Here's how the part is built. I have some questions about the finished solid (model axes, mm). Coordinates: 2 decimals unless noted, no trailing zeros. Write each loop counter-clockwise with the first axis right and the second up, starting at its lowest first coordinate (ties: lowest second). Pieces come first, ordered by that corner, then holes. Notation, with made-up numbers: (33.25, 80) -> (85.25, 80) arc R27 cw to (85.25, 103) -> close; hole circle Ø8 at (4, -9). An arc over 180 degrees is marked (long way). Use a Markdown table: item, result. Add a question column.
Item 1: If I drill on line 1 along Y through (x, z) = (0, 18.5); line 2 along X through (y, z) = (-3, 7.75); line 3 along X through (y, z) = (6, 2), over which ranges is the centre line in solid material (lowest first)? Write a range as from..to.
Item 2: Imagine slicing it at C-C, the plane z = 3. Write out the boundary of the cut face in (x, y).
Item 3: Will these pins go through, and if not, where does the flat tip stop? pin 1 Ø2 at (x, z) = (-12, 12.5) entering from +Y; pin 2 Ø9 at (x, y) = (0, 0) entering from +Z.
Item 4: If we mould it in two halves opening along X, with no side actions, what happens to faces 1 (the flat face through (15, 0, 12)), 2 (the flat face through (-15, 0, 12)), 3 (the flat face through (6, -5, 0)), 4 (the cylindrical face through (-7.493, 0.33, 12.325))? For each: pulls with the +X half, pulls with the -X half, needs draft (parallel to the pull), parting line crosses it, or undercut.
Item 5: Imagine slicing it at B-B, the plane y = 0. Write out the boundary of the cut face in (x, z), and give its area (3 significant figures).
Item 6: Imagine slicing it at A-A, the plane x = 0. Write out the boundary of the cut face in (y, z).
Item 7: Imagine slicing it at D-D, the plane y = -22. Write out the boundary of the cut face in (x, z).
```python
from build123d import *

# Parameters (mm, degrees)
F0_W     = 30
F0_H     = 50
F0_R     = 7.5
F1_DEPTH = 25
F2_SIZE  = 5


with BuildPart() as f1:
    # F0 (on Top) → F1 (new body)
    with BuildSketch(Plane.XY):
        Rectangle(F0_W, F0_H)
        Circle(F0_R, mode=Mode.SUBTRACT)
    extrude(amount=F1_DEPTH)

    # F2
    f2_edges = [f1.edges().sort_by_distance(p)[0] for p in [
        (15, -25, 12.5),
        (-15, -25, 12.5),
        (15, 25, 12.5),
        (-15, 25, 12.5),
    ]]
    chamfer(f2_edges, length=F2_SIZE)


solid = f1.part
```
Ans:
| question | item | result |
|---|---|---|
| 1 | line 1 | y = -25..-7.5, 7.5..25 |
| 1 | line 2 | x = -15..-6.87, 6.87..15 |
| 1 | line 3 | x = -15..-4.5, 4.5..15 |
| 2 | outline | (-15, -20) -> (-10, -25) -> (10, -25) -> (15, -20) -> (15, 20) -> (10, 25) -> (-10, 25) -> (-15, 20) -> close; hole circle Ø15 at (0, 0) |
| 3 | pin 1 | stops at y = 24 |
| 3 | pin 2 | passes through |
| 4 | face 1 | pulls with the +X half |
| 4 | face 2 | pulls with the -X half |
| 4 | face 3 | needs draft |
| 4 | face 4 | undercut |
| 5 | outline | (-15, 0) -> (-7.5, 0) -> (-7.5, 25) -> (-15, 25) -> close; (7.5, 0) -> (15, 0) -> (15, 25) -> (7.5, 25) -> close |
| 5 | area | 375 mm^2 |
| 6 | outline | (-25, 0) -> (-7.5, 0) -> (-7.5, 25) -> (-25, 25) -> close; (7.5, 0) -> (25, 0) -> (25, 25) -> (7.5, 25) -> close |
| 7 | outline | (-13, 0) -> (13, 0) -> (13, 25) -> (-13, 25) -> close |
